from build123d import *

# Parameters (mm, degrees)
SKETCH1_W             = 25.875
SKETCH1_H             = 31.75
BOSS_EXTRUDE1_DEPTH   = 6.35
SKETCH1_4_OUTSIDE_W   = 36.165
SKETCH1_4_OUTSIDE_H   = 42.04
SKETCH1_4_OUTSIDE_W_2 = 25.875
SKETCH1_4_OUTSIDE_H_2 = 31.75
SKETCH1_4_OUTSIDE_R   = 2.551011908
CUT_EXTRUDE3_DEPTH    = 7.35


with BuildPart() as part:
    # Sketch1 → Boss-Extrude1 (new body)
    with BuildSketch(Plane.XY):
        with Locations((-35.541307617, 35.200886597)):
            Rectangle(SKETCH1_W, SKETCH1_H)
    extrude(amount=BOSS_EXTRUDE1_DEPTH)

    # Sketch1_4 outside → Cut-Extrude3 (cut, through all)
    with BuildSketch(Plane.XY):
        with Locations((-35.5415, 35.201)):
            Rectangle(SKETCH1_4_OUTSIDE_W, SKETCH1_4_OUTSIDE_H)
        with Locations((-35.541307617, 35.200886597)):
            Rectangle(SKETCH1_4_OUTSIDE_W_2, SKETCH1_4_OUTSIDE_H_2, mode=Mode.SUBTRACT)
        with Locations((-32.603807617, 38.375886597)):
            Circle(SKETCH1_4_OUTSIDE_R)
    extrude(amount=CUT_EXTRUDE3_DEPTH, mode=Mode.SUBTRACT)


solid = part.part
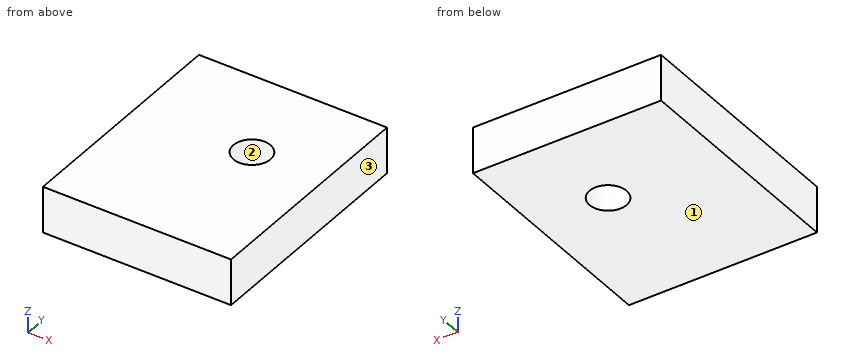
Could you check a few things on this model? Use its own coordinates, in mm. Face numbers are marked on the shaded views. Round coordinates to 2 decimals unless told otherwise and drop trailing zeros. Write each loop counter-clockwise with the first axis right and the second up, starting at its lowest first coordinate (ties: lowest second). Pieces come first, ordered by that corner, then holes. Notation, with made-up numbers: (-22, -35.75) - (-14, -35.75) arc R19 ccw to (-14, 1.25) - close; hole circle Ø3 at (2.5, -12.75). An arc over 180 degrees is marked (long way). Use a Markdown table: item, result.
Q1. I want a section at C-C (x = -30.5). List the corners of the cut face in (y, z) for me, plus the area to 3 significant figures.
Output values:
| item | result |
|---|---|
| outline | (19.33, 0) - (36.93, 0) - (36.93, 6.35) - (19.33, 6.35) - close; (39.82, 0) - (51.08, 0) - (51.08, 6.35) - (39.82, 6.35) - close |
| area | 183 mm2 |
Q2. I want a section at B-B (z = 1.75). List the corners of the cut face in (x, y) for me.
Output values:
| item | result |
|---|---|
| outline | (-48.48, 19.33) - (-22.6, 19.33) - (-22.6, 51.08) - (-48.48, 51.08) - close; hole circle Ø5.1 at (-32.6, 38.38) |
Q3. Please list where these lines run through material, in increasing order: L1, parallel to Y at x = -34.75, z = 4.75; L2, parallel to X at y = 37, z = 1.25; L3, parallel to X at y = 38, z = 1.75.
Output values:
| item | result |
|---|---|
| L1 | 19.33 to 37, 39.75 to 51.08 |
| L2 | -48.48 to -34.75, -30.46 to -22.6 |
| L3 | -48.48 to -35.13, -30.08 to -22.6 |
Q4. I want a section at A-A (x = -34.25). List the corners of the cut face in (y, z) for me.
Output values:
| item | result |
|---|---|
| outline | (19.33, 0) - (36.43, 0) - (36.43, 6.35) - (19.33, 6.35) - close; (40.32, 0) - (51.08, 0) - (51.08, 6.35) - (40.32, 6.35) - close |
Q5. Thinking about a two-plate mould opening in X: for the marked faces 1, 2 and 3, which applies, released by +X, released by -X, zero draft, split by the parting line, or undercut?
Output values:
| item | result |
|---|---|
| face 1 | zero draft |
| face 2 | undercut |
| face 3 | released by +X |
